from build123d import *

# Parameters (mm, degrees)
SKETCH1_W           = 16
SKETCH1_H           = 16
SKETCH1_W_2         = 14
SKETCH1_H_2         = 14
BOSS_EXTRUDE1_DEPTH = 198.575758147
SKETCH2_R           = 3.75
SKETCH2_R_2         = 3
SKETCH2_R_3         = 1.4
SKETCH2_R_4         = 1.6
CUT_EXTRUDE1_DEPTH  = 200.3798679


with BuildPart() as part:
    # Sketch1 → Boss-Extrude1 (new body)
    with BuildSketch(Plane.XY):
        Rectangle(SKETCH1_W, SKETCH1_H)
        Rectangle(SKETCH1_W_2, SKETCH1_H_2, mode=Mode.SUBTRACT)
    extrude(amount=BOSS_EXTRUDE1_DEPTH)

    # Sketch2 → Cut-Extrude1 (cut, through all)
    with BuildSketch(Plane(origin=(0, 8, 0), x_dir=(1, 0, 0), z_dir=(0, 1, 0))):
        with Locations(Location((0, -9.5, 0), (0, 0, 270))):
            Circle(SKETCH2_R)
        with Locations(Location((0, -20.5, 0), (0, 0, 270))):
            Circle(SKETCH2_R_2)
        with Locations(Location((0, -170, 0), (0, 0, 270))):
            Circle(SKETCH2_R_3)
        with Locations(Location((0, -183.5, 0), (0, 0, 270))):
            Circle(SKETCH2_R_4)
    extrude(amount=-CUT_EXTRUDE1_DEPTH, mode=Mode.SUBTRACT)


solid = part.part
Design review of the part built by this model. Coordinates are the model's own, in mm. A direction names the side the tool comes from. Give positions to 0.01 mm unless a question says otherwise; leave off trailing zeros. Loops run counter-clockwise (first coordinate to the right, second up) from the corner with the lowest first, then second, coordinate; pieces in that order, holes last. Notation, with made-up numbers: M 60.5,20.5 L 100.5,20.5 A8 cw 100.5,27.5 Z; hole C 66,19.5 d6. An arc over 180 degrees is marked long. One line per question, with ' | ' between items. Start each with the question number.
1. Add section B-B (z = 94). Write out the cut boundary in (x, y).
2. Add section C-C (z = 20.5). Write out the cut boundary in (x, y), plus the area to 3 significant figures.
3. Add section A-A (y = -2.75). Write out the cut boundary in (x, z), plus the area to 3 significant figures.
4. To check wall thickness, follow L1, parallel to X at y = 7.35, z = 9.5; L2, parallel to X at y = -7.55, z = 20.5; L3, parallel to Y at x = 6.5, z = 161.5. State the ranges of each line that lie inside material, in increasing order.
5. The part is to be moulded in two halves that separate along Y. For faces 3 (the face through (8, 0, 98)), 4 (the face through (0, -8, 98)), 5 (the face through (0, -7, 98)), say which applies: released by +Y, released by -Y, zero draft, split by the parting line, or undercut.
6. For faces 1 (the face through (0.1, -7.5, 17.5)), 2 (the face through (0, 7, 98)), list the 3-axis set-ups (+Z, -Z, +X, -X, +Y, -Y) from which the entire face can be reached by the end or side of a thin tool; tool diameter is ignored.
7. Add section D-D (z = 183.5). Write out the cut boundary in (x, y), plus the area to 3 significant figures.
Worked out:
1) outline: M -8,-8 L 8,-8 L 8,8 L -8,8 Z; hole M -7,-7 L 7,-7 L 7,7 L -7,7 Z
2) outline: M -8,-8 L -3,-8 L -3,-7 L -7,-7 L -7,7 L -3,7 L -3,8 L -8,8 Z; M 3,-8 L 8,-8 L 8,8 L 3,8 L 3,7 L 7,7 L 7,-7 L 3,-7 Z | area: 48.0 mm²
3) outline: M -8,0 L -7,0 L -7,198.58 L -8,198.58 Z; M 7,0 L 8,0 L 8,198.58 L 7,198.58 Z | area: 397 mm²
4) L1: x = -8 to -3.75, 3.75 to 8 | L2: x = -8 to -3, 3 to 8 | L3: y = -8 to -7, 7 to 8
5) face 3: zero draft | face 4: released by -Y | face 5: undercut
6) face 1: +Y, -Y | face 2: +Z, -Z
7) outline: M -8,-8 L -1.6,-8 L -1.6,-7 L -7,-7 L -7,7 L -1.6,7 L -1.6,8 L -8,8 Z; M 1.6,-8 L 8,-8 L 8,8 L 1.6,8 L 1.6,7 L 7,7 L 7,-7 L 1.6,-7 Z | area: 53.6 mm²
